Could you check a few things on this drawing? It's one solid part, dimensions in mm from its lowest x, y, z. Give positions to 0.01 mm unless a question says otherwise; leave off trailing zeros. Write each loop counter-clockwise with the first axis right and the second up, starting at its lowest first coordinate (ties: lowest second). Pieces come first, ordered by that corner, then holes. Notation, with made-up numbers: M 19,41 L 78,41 A8 ccw 78,48 Z; hole C 51,42.25 d4. An arc over 180 degrees is marked long. Use CSV: the item, a comma, the result in double quotes. Start each with the question number.
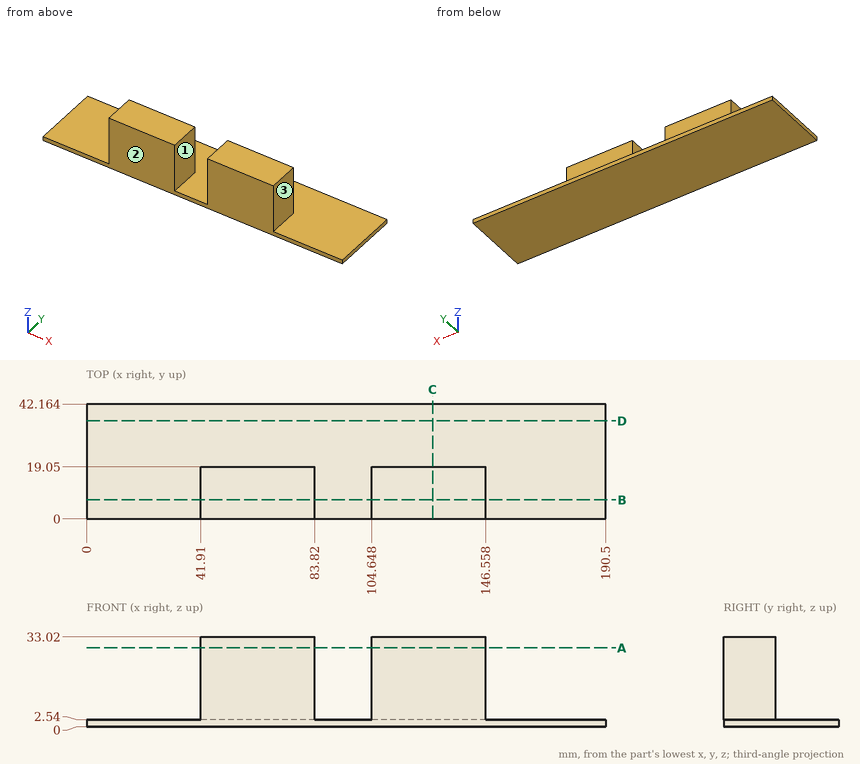
(1) I want a section at A-A (z = 29). Write out the boundary of the cut face in (x, y), and give its area (3 significant figures).
(2) Will these pins go through, and if not, where does the flat tip stop? pin 1 Ø15 at (y, z) = (8.5, 22) entering from +X; pin 2 Ø12 at (x, z) = (121, 18) entering from +Y; pin 3 Ø2 at (y, z) = (18.5, 6) entering from -X.
(3) I want a section at D-D (y = 36). Write out the boundary of the cut face in (x, z), and give its area (3 significant figures).
(4) I want a section at B-B (y = 7). Write out the boundary of the cut face in (x, z), and give its area (3 significant figures).
(5) Thinking about a two-plate mould opening in X: for the marked faces 1, 2 and 3, which applies, released by +X, released by -X, zero draft, split by the parting line, or undercut?
(6) I want a section at C-C (x = 127). Write out the boundary of the cut face in (y, z).
(7) Please list where these lines run through material, in increasing order: L1, parallel to X at y = 12, z = 28; L2, parallel to Z at x = 14, y = 15.5; L3, parallel to Y at x = 79.5, z = 5.5. Write a range as [from, to].
Geometry results:
1,outline,"M 41.91,0 L 83.82,0 L 83.82,19.05 L 41.91,19.05 Z; M 104.65,0 L 146.56,0 L 146.56,19.05 L 104.65,19.05 Z"
1,area,"1,600 mm2"
2,pin 1,"stops at x = 146.56"
2,pin 2,"stops at y = 19.05"
2,pin 3,"stops at x = 41.91"
3,outline,"M 0,0 L 190.5,0 L 190.5,2.54 L 0,2.54 Z"
3,area,"484 mm2"
4,outline,"M 0,0 L 190.5,0 L 190.5,2.54 L 146.56,2.54 L 146.56,33.02 L 104.65,33.02 L 104.65,2.54 L 83.82,2.54 L 83.82,33.02 L 41.91,33.02 L 41.91,2.54 L 0,2.54 Z"
4,area,"3,040 mm2"
5,face 1,"undercut"
5,face 2,"zero draft"
5,face 3,"released by +X"
6,outline,"M 0,0 L 42.16,0 L 42.16,2.54 L 19.05,2.54 L 19.05,33.02 L 0,33.02 Z"
7,L1,"x = [41.91, 83.82], [104.65, 146.56]"
7,L2,"z = [0, 2.54]"
7,L3,"y = [0, 19.05]"
